Can you work these out from the model? Positions are in its coordinate system, mm. Face numbers are marked on the shaded views. Give positions to 0.01 mm unless a question says otherwise; leave off trailing zeros. Loops run counter-clockwise (first coordinate to the right, second up) from the corner with the lowest first, then second, coordinate; pieces in that order, holes last.
from build123d import *

# Parameters (mm, degrees)
SKETCH_1_W          = 80
SKETCH_1_H          = 40
EXTRUDE_1_DEPTH     = 10
SKETCH_2_R          = 5
CUT_EXTRUDE_1_DEPTH = 91


with BuildPart() as part:
    # 草图1 → 凸台-拉伸1 (new body)
    with BuildSketch(Plane.XY.offset(-5)):
        with Locations((40, 20)):
            Rectangle(SKETCH_1_W, SKETCH_1_H)
    extrude(amount=EXTRUDE_1_DEPTH)

    # 草图2 → 切除-拉伸1 (cut, through all)
    with BuildSketch(Plane.XY.offset(5)):
        with Locations((20, 20)):
            Circle(SKETCH_2_R)
        with Locations((60, 20)):
            Circle(SKETCH_2_R)
    extrude(amount=-CUT_EXTRUDE_1_DEPTH, mode=Mode.SUBTRACT)


solid = part.part
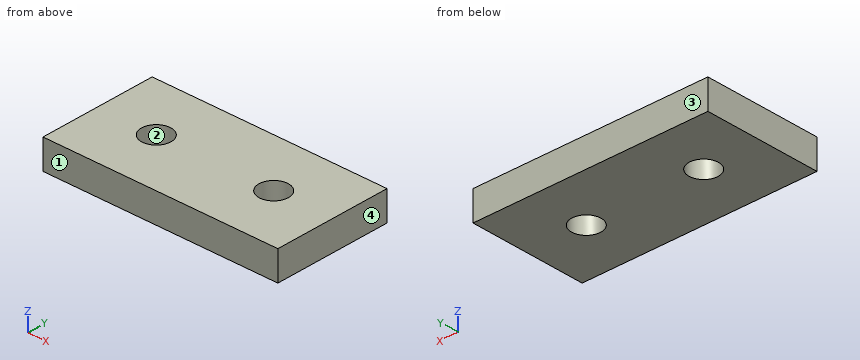
(1) Suppose I cut it at A-A on x = 20. List the corners of the cut face in (y, z) for me.
Returned:
outline: (0, -5) - (15, -5) - (15, 5) - (0, 5) - close; (25, -5) - (40, -5) - (40, 5) - (25, 5) - close
(2) Suppose I cut it at C-C on z = 2.5. List the corners of the cut face in (x, y) for me, plus the area to 3 significant figures.
Returned:
outline: (0, 0) - (80, 0) - (80, 40) - (0, 40) - close; hole circle Ø10 at (20, 20); hole circle Ø10 at (60, 20)
area: 3,040 mm2
(3) Please list where these lines run through material, in increasing order: probe 1 along Y at (x, z) = (20, 1.75); probe 2 along X at (y, z) = (21, -1.25); probe 3 along X at (y, z) = (23, -0.25).
Returned:
probe 1: y = 0 to 15, 25 to 40
probe 2: x = 0 to 15.1, 24.9 to 55.1, 64.9 to 80
probe 3: x = 0 to 16, 24 to 56, 64 to 80
(4) Thinking about a two-plate mould opening in Y: for the marked faces 1, 2, 3 and 4, which applies, pulls with the +Y half, pulls with the -Y half, needs draft (parallel to the pull), parting line crosses it, or undercut?
Returned:
face 1: pulls with the -Y half
face 2: undercut
face 3: pulls with the +Y half
face 4: needs draft
(5) Suppose I cut it at B-B on y = 20. List the corners of the cut face in (x, z) for me.
Returned:
outline: (0, -5) - (15, -5) - (15, 5) - (0, 5) - close; (25, -5) - (55, -5) - (55, 5) - (25, 5) - close; (65, -5) - (80, -5) - (80, 5) - (65, 5) - close
